from build123d import *

# Parameters (mm, degrees)
SKETCH1_R           = 19.04
BOSS_EXTRUDE1_DEPTH = 558.8


with BuildPart() as part:
    # Sketch1 → Boss-Extrude1 (new body)
    with BuildSketch(Plane.XY):
        Circle(SKETCH1_R)
        with BuildLine():
            Line((10.08336557, 10.867675179), (12.467953414, 12.244417612))
            ThreePointArc((12.467953414, 12.244417612), (15.133793931, 8.7375), (16.837953414, 4.675355583))
            Line((16.837953414, 4.675355583), (14.45336557, 3.29861315))
            ThreePointArc((14.45336557, 3.29861315), (14.825, 0), (14.45336557, -3.29861315))
            Line((14.45336557, -3.29861315), (16.837953414, -4.675355583))
            ThreePointArc((16.837953414, -4.675355583), (15.133793931, -8.7375), (12.467953414, -12.244417612))
            Line((12.467953414, -12.244417612), (10.08336557, -10.867675179))
            ThreePointArc((10.08336557, -10.867675179), (7.4125, -12.838826611), (4.37, -14.166288328))
            Line((4.37, -14.166288328), (4.37, -16.919773196))
            ThreePointArc((4.37, -16.919773196), (0, -17.475), (-4.37, -16.919773196))
            Line((-4.37, -16.919773196), (-4.37, -14.166288328))
            ThreePointArc((-4.37, -14.166288328), (-7.4125, -12.838826611), (-10.08336557, -10.867675179))
            Line((-10.08336557, -10.867675179), (-12.467953414, -12.244417612))
            ThreePointArc((-12.467953414, -12.244417612), (-15.133793931, -8.7375), (-16.837953414, -4.675355583))
            Line((-16.837953414, -4.675355583), (-14.45336557, -3.29861315))
            ThreePointArc((-14.45336557, -3.29861315), (-14.825, 0), (-14.45336557, 3.29861315))
            Line((-14.45336557, 3.29861315), (-16.837953414, 4.675355583))
            ThreePointArc((-16.837953414, 4.675355583), (-15.133793931, 8.7375), (-12.467953414, 12.244417612))
            Line((-12.467953414, 12.244417612), (-10.08336557, 10.867675179))
            ThreePointArc((-10.08336557, 10.867675179), (-7.4125, 12.838826611), (-4.37, 14.166288328))
            Line((-4.37, 14.166288328), (-4.37, 16.919773196))
            ThreePointArc((-4.37, 16.919773196), (0, 17.475), (4.37, 16.919773196))
            Line((4.37, 16.919773196), (4.37, 14.166288328))
            ThreePointArc((4.37, 14.166288328), (7.4125, 12.838826611), (10.08336557, 10.867675179))
        make_face(mode=Mode.SUBTRACT)
    extrude(amount=BOSS_EXTRUDE1_DEPTH)


solid = part.part
Work out the finished part from the listing and answer in its coordinate system (mm). A direction names the side the tool comes from. Give positions to 0.01 mm unless a question says otherwise; leave off trailing zeros. Loops run counter-clockwise (first coordinate to the right, second up) from the corner with the lowest first, then second, coordinate; pieces in that order, holes last. Notation, with made-up numbers: (76.25, 8) -> (80.25, 8) arc R10 cw to (80.25, 26) -> close; hole circle Ø7 at (64.5, 77). An arc over 180 degrees is marked (long way). Use a Markdown table: item, result. Add a question column.
1) Each of these flat-tipped pins is pushed along its axis until it touches: P1, Ø3, axis at y = -15.5, z = 381, coming from the +X side; P2, Ø3, axis at x = 2.5, z = 101, coming from the +Y side; P3, Ø1.5, axis at y = -8, z = 324, coming from the -X side. Where does it stop, or does it pass through?
2) The part is cut by section A-A, the plane z = 459. Determine the outline of the cut face in (x, y) (3 decimals), plus the area to 3 significant figures.
3) Which of the six approach directions +Z, -Z, +X, -X, +Y, -Y give full straight-line access (tool end or side, diameter ignored) to faces 4 (the cylindrical face through (-0.062, 17.475, 275.488)), 5 (the flat face through (9.8, 11.4, 0))?
4) Consider line 1 along Y through (x, z) = (15, 418); line 2 along X through (y, z) = (-0.5, 292); line 3 along X through (y, z) = (11.5, 349.5). Determine where each line is inside the solid, lowest interval first.
5) For a pull along X with two mould halves and no side action, classify faces 1 (the cylindrical face through (-4.127, -18.587, 275.488)), 2 (the flat face through (9.8, 11.4, 558.8)), 3 (the cylindrical face through (0.062, -17.475, 275.488)) as +X half, -X half, draft (parallel to the pull), parting line (faces both ways), or undercut.
Reported:
| question | item | result |
|---|---|---|
| 1 | P1 | stops at x = 12.9 |
| 1 | P2 | stops at y = 19.01 |
| 1 | P3 | stops at x = -17.61 |
| 2 | outline | circle Ø38.08 at (0, 0); hole (-16.838, -4.675) arc R17.475 ccw to (-12.468, -12.244) -> (-10.083, -10.868) arc R14.825 ccw to (-4.37, -14.166) -> (-4.37, -16.92) arc R17.475 ccw to (4.37, -16.92) -> (4.37, -14.166) arc R14.825 ccw to (10.083, -10.868) -> (12.468, -12.244) arc R17.475 ccw to (16.838, -4.675) -> (14.453, -3.299) arc R14.825 ccw to (14.453, 3.299) -> (16.838, 4.675) arc R17.475 ccw to (12.468, 12.244) -> (10.083, 10.868) arc R14.825 ccw to (4.37, 14.166) -> (4.37, 16.92) arc R17.475 ccw to (-4.37, 16.92) -> (-4.37, 14.166) arc R14.825 ccw to (-10.083, 10.868) -> (-12.468, 12.244) arc R17.475 ccw to (-16.838, 4.675) -> (-14.453, 3.299) arc R14.825 ccw to (-14.453, -3.299) -> close |
| 2 | area | 308 mm^2 |
| 3 | face 4 | +Z, -Z |
| 3 | face 5 | -Z, +X, -X, +Y, -Y |
| 4 | line 1 | y = -11.73 to -8.97, -3.61 to 3.61, 8.97 to 11.73 |
| 4 | line 2 | x = -19.03 to -14.82, 14.82 to 19.03 |
| 4 | line 3 | x = -15.17 to -13.16, -11.18 to -9.36, 9.36 to 11.18, 13.16 to 15.17 |
| 5 | face 1 | parting line |
| 5 | face 2 | draft |
| 5 | face 3 | undercut |
